```python
from build123d import *

# Parameters (mm, degrees)
SKETCH1_W           = 62.23
SKETCH1_H           = 20.066
BOSS_EXTRUDE1_DEPTH = 25.4
BOSS_EXTRUDE2_DEPTH = 25.4
SKETCH4_W           = 8.89
SKETCH4_H           = 6.35
BOSS_EXTRUDE3_DEPTH = 25.4
SKETCH5_R           = 2.54
CUT_EXTRUDE1_DEPTH  = 7.35
SKETCH10_W          = 41.3004
SKETCH10_H          = 20.066
CUT_EXTRUDE6_DEPTH  = 19.05
SKETCH11_R          = 2.286
CUT_EXTRUDE7_DEPTH  = 26.4


with BuildPart() as part:
    # Sketch1 → Boss-Extrude1 (new body)
    with BuildSketch(Plane.XY):
        with Locations((3812.36685564, 1.533)):
            Rectangle(SKETCH1_W, SKETCH1_H)
    extrude(amount=BOSS_EXTRUDE1_DEPTH)

    # Sketch3 → Boss-Extrude2 (add)
    with BuildSketch(Plane(origin=(0, 11.566, 0), x_dir=(1, 0, 0), z_dir=(0, 1, 0))):
        Polygon((3831.44225564, 0), (3831.44225564, -6.35), (3840.33225564, -6.35), (3840.33225564, -25.4), (3843.48185564, -25.4), (3843.48185564, 0), align=None)
    extrude(amount=BOSS_EXTRUDE2_DEPTH)

    # Sketch4 → Boss-Extrude3 (add)
    with BuildSketch(Plane(origin=(0, 11.566, 0), x_dir=(1, 0, 0), z_dir=(0, 1, 0))):
        with Locations((3785.69685564, -3.175)):
            Rectangle(SKETCH4_W, SKETCH4_H)
    extrude(amount=BOSS_EXTRUDE3_DEPTH)

    # Sketch5 → Cut-Extrude1 (cut, through all)
    with BuildSketch(Plane.XY.offset(6.35)):
        with Locations((3835.76025564, 30.616)):
            Circle(SKETCH5_R)
        with Locations((3835.76025564, 20.71)):
            Circle(SKETCH5_R)
        with Locations((3786.23025564, 20.71)):
            Circle(SKETCH5_R)
        with Locations((3786.23025564, 30.616)):
            Circle(SKETCH5_R)
    extrude(amount=-CUT_EXTRUDE1_DEPTH, mode=Mode.SUBTRACT)

    # Sketch10 → Cut-Extrude6 (cut)
    with BuildSketch(Plane(origin=(0, 0, 0), x_dir=(-1, 0, 0), z_dir=(0, 0, -1))):
        with Locations((-3810.79205564, 1.533)):
            Rectangle(SKETCH10_W, SKETCH10_H)
    extrude(amount=-CUT_EXTRUDE6_DEPTH, mode=Mode.SUBTRACT)

    # Sketch11 → Cut-Extrude7 (cut, through all)
    with BuildSketch(Plane.XY.offset(25.4)):
        with Locations((3799.66685564, 1.533)):
            Circle(SKETCH11_R)
        with Locations((3825.06685564, 1.533)):
            Circle(SKETCH11_R)
    extrude(amount=-CUT_EXTRUDE7_DEPTH, mode=Mode.SUBTRACT)


solid = part.part
```
Geometry: final body of the model. Coordinates: model frame, mm. A direction names the side the tool comes from. Round coordinates to 2 decimals unless told otherwise and drop trailing zeros. Order: outer loops, then holes, each group sorted by start corner. A loop starts at its lowest first (then second) coordinate and runs counter-clockwise, first axis right, second up. Notation, with made-up numbers: M -20.5,45.5 L -1.5,45.5 A33 cw -1.5,75.5 Z; hole C -37,0.5 d3. An arc over 180 degrees is marked long. One line per item, written item: value.
(1) Line query: probe 1 along X at (y, z) = (-3, 16.5); probe 2 along X at (y, z) = (31.5, 7); probe 3 along Z at (x, y) = (3832, 12.5). Output: solid intervals per line, ascending. Write a range as [from, to].
Result sheet:
probe 1: [3781.25, 3790.14], [3831.44, 3843.48]
probe 2: [3840.33, 3843.48]
probe 3: [0, 6.35]
(2) Cut plane A-A (z = 7). Return the cut outline in (x, y), and give its area (3 significant figures).
Result sheet:
outline: M 3781.25,-8.5 L 3790.14,-8.5 L 3790.14,11.57 L 3781.25,11.57 Z; M 3831.44,-8.5 L 3843.48,-8.5 L 3843.48,36.97 L 3840.33,36.97 L 3840.33,11.57 L 3831.44,11.57 Z
area: 500 mm2
(3) Pin query (flat end, axial travel): P1, Ø3, axis at x = 3835.76, y = 30.62, coming from the -Z side; P2, Ø10, axis at x = 3808.5, y = 3.5, coming from the -Z side. Return the tip coordinate at first contact, or that it passes through.
Result sheet:
P1: through
P2: z = 19.05
(4) Cut plane C-C (x = 3834.5). Return the cut outline in (y, z).
Result sheet:
outline: M -8.5,0 L 18.5,0 L 18.5,6.35 L 11.57,6.35 L 11.57,25.4 L -8.5,25.4 Z; M 22.92,0 L 28.41,0 L 28.41,6.35 L 22.92,6.35 Z; M 32.82,0 L 36.97,0 L 36.97,6.35 L 32.82,6.35 Z
(5) Cut plane D-D (y = 15). Return the cut outline in (x, z), and give its area (3 significant figures).
Result sheet:
outline: M 3781.25,0 L 3790.14,0 L 3790.14,6.35 L 3781.25,6.35 Z; M 3831.44,0 L 3843.48,0 L 3843.48,25.4 L 3840.33,25.4 L 3840.33,6.35 L 3831.44,6.35 Z
area: 193 mm2
(6) Cut plane B-B (y = 20.71). Return the cut outline in (x, z).
Result sheet:
outline: M 3781.25,0 L 3783.69,0 L 3783.69,6.35 L 3781.25,6.35 Z; M 3788.77,0 L 3790.14,0 L 3790.14,6.35 L 3788.77,6.35 Z; M 3831.44,0 L 3833.22,0 L 3833.22,6.35 L 3831.44,6.35 Z; M 3838.3,0 L 3843.48,0 L 3843.48,25.4 L 3840.33,25.4 L 3840.33,6.35 L 3838.3,6.35 Z
(7) Pull-direction query (X, two-part tool) for faces 4 (the flat face through (3841, 36.966, 7)), 5 (the cylindrical face through (3797.383, 1.634, 22.269)), 6 (the flat face through (3843.482, 14, 13)), 7 (the flat face through (3811, 2, 19.05)); classes: pulls with the +X half, pulls with the -X half, needs draft (parallel to the pull), parting line crosses it, or undercut.
Result sheet:
face 4: needs draft
face 5: undercut
face 6: pulls with the +X half
face 7: undercut
(8) Reachability of faces 1 (the flat face through (3831.442, 9, 7)), 2 (the flat face through (3836, 24, 6.35)), 3 (the flat face through (3837, 14, 0)) from +Z, -Z, +X, -X, +Y, -Y: full face, straight path, thin tool, end or side. Return the list, or none.
Result sheet:
face 1: -Z, +Y, -Y
face 2: +Z, -X, +Y
face 3: -Z, +X, -X, +Y, -Y
